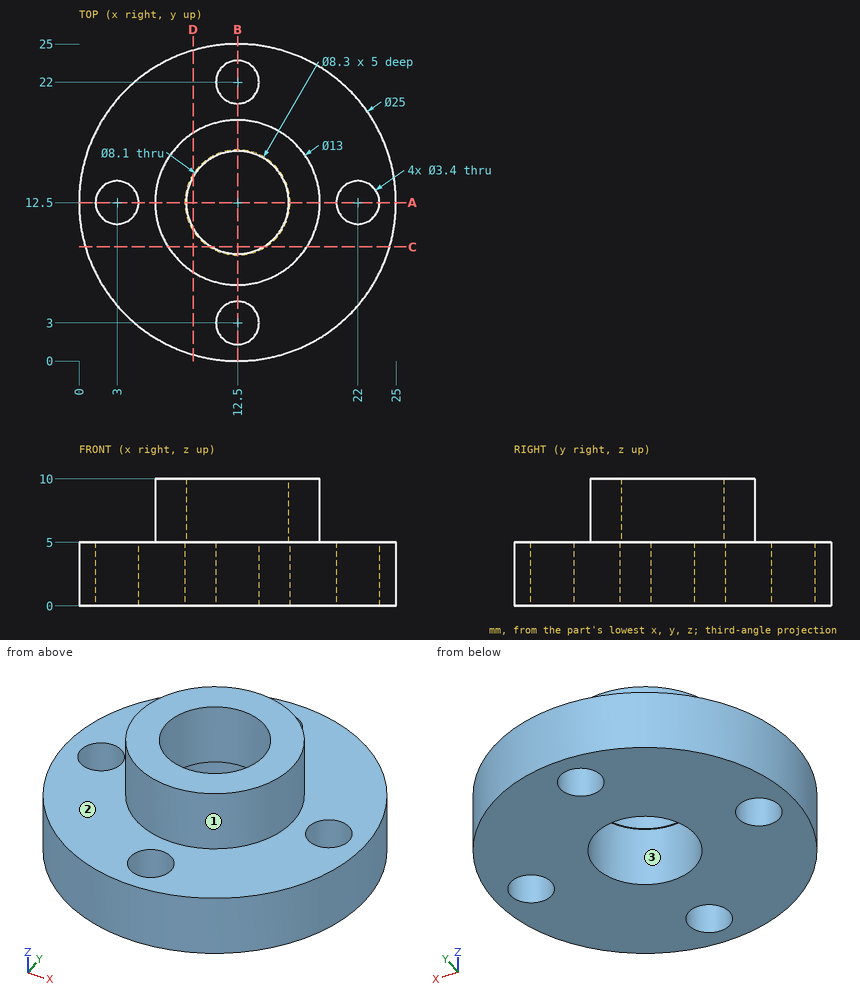
Source: three-view drawing plus pictorial views. Frame: mm from the lowest corner of the part. Coordinates: 2 decimals unless noted, no trailing zeros. Write each loop counter-clockwise with the first axis right and the second up, starting at its lowest first coordinate (ties: lowest second). Pieces come first, ordered by that corner, then holes. Notation, with made-up numbers: (1.5, 44) - (14.5, 44) arc R10 cw to (14.5, 60) - close; hole circle Ø9 at (38, 41). An arc over 180 degrees is marked (long way). Answer as a JSON object with one key per item and string values.
Q1. Section query A-A, the plane y = 12.5. Output: boundary loops of the cut face in (x, z).
Ans:
{"outline": "(0, 0) - (1.3, 0) - (1.3, 5) - (0, 5) - close; (4.7, 0) - (8.35, 0) - (8.35, 5) - (8.45, 5) - (8.45, 10) - (6, 10) - (6, 5) - (4.7, 5) - close; (16.55, 5) - (16.65, 5) - (16.65, 0) - (20.3, 0) - (20.3, 5) - (19, 5) - (19, 10) - (16.55, 10) - close; (23.7, 0) - (25, 0) - (25, 5) - (23.7, 5) - close"}
Q2. Section query C-C, the plane y = 9. Output: boundary loops of the cut face in (x, z), plus the area to 3 significant figures.
Ans:
{"outline": "(0.5, 0) - (10.27, 0) - (10.27, 5) - (10.46, 5) - (10.46, 10) - (7.02, 10) - (7.02, 5) - (0.5, 5) - close; (14.54, 5) - (14.73, 5) - (14.73, 0) - (24.5, 0) - (24.5, 5) - (17.98, 5) - (17.98, 10) - (14.54, 10) - close", "area": "132 mm2"}
Q3. First-contact query: pin 1 Ø2.5 at (x, y) = (11.5, 11.5) entering from -Z; pin 2 Ø1.5 at (y, z) = (7.5, 5) entering from +X; pin 3 Ø5.5 at (x, y) = (22, 12.5) entering from +Z; pin 4 Ø6 at (x, z) = (19.5, 6) entering from +Y. Flat tips, straight axial feed; report the tip coordinate or a pass-through.
Ans:
{"pin 1": "passes through", "pin 2": "stops at x = 24.26", "pin 3": "stops at z = 5", "pin 4": "stops at y = 24.28"}
Q4. Material intervals for line 1 (Y direction, x = 12.5, z = 3.65); line 2 (Y direction, x = 12.5, z = 6.3); line 3 (Y direction, x = 4.25, z = 2.75), sorted ascending. Write a range as [from, to].
Ans:
{"line 1": "y = [0, 1.3], [4.7, 8.35], [16.65, 20.3], [23.7, 25]", "line 2": "y = [6, 8.45], [16.55, 19]", "line 3": "y = [3.11, 11.35], [13.65, 21.89]"}
Q5. Draft query along Y for the marked faces 1, 2 and 3. Return one class per face: released by +Y, released by -Y, zero draft, split by the parting line, or undercut.
Ans:
{"face 1": "split by the parting line", "face 2": "zero draft", "face 3": "undercut"}
